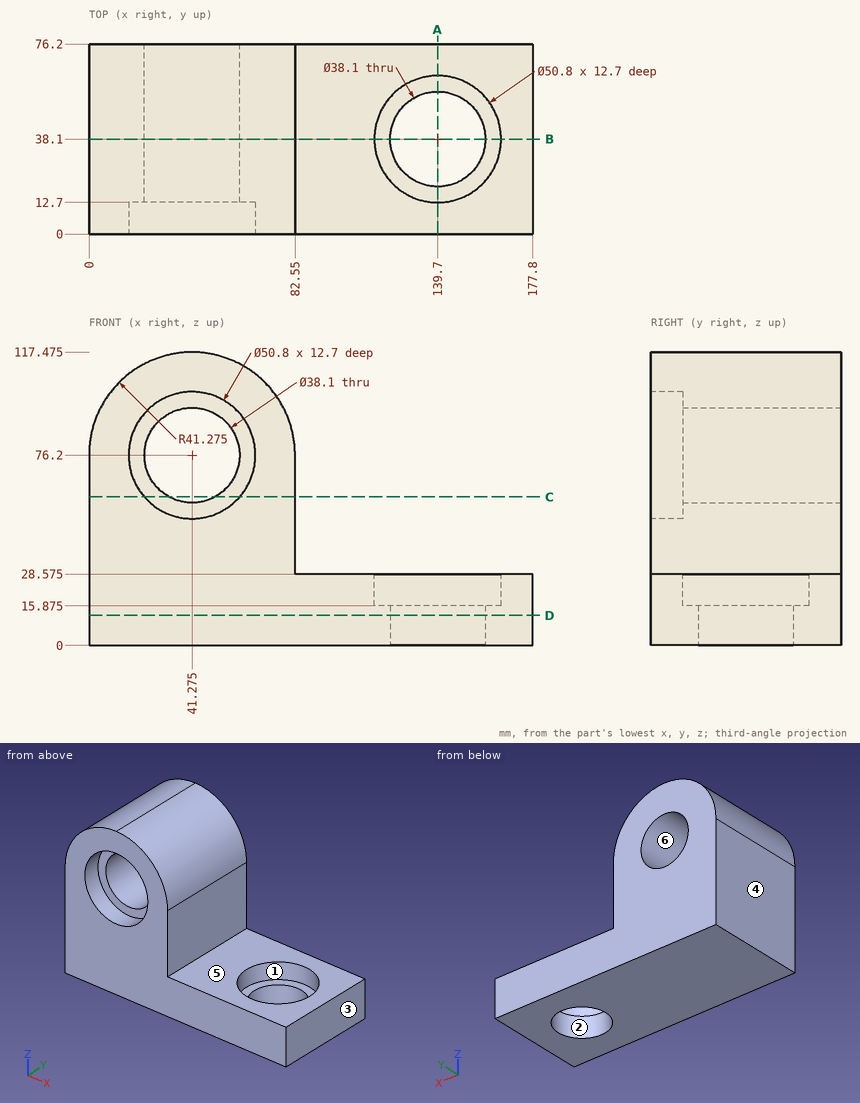
Print and shaded views of the part. All mm, measured from the part's lowest x, y and z. A direction names the side the tool comes from. Coordinates: 2 decimals unless noted, no trailing zeros. Loops run counter-clockwise (first coordinate to the right, second up) from the corner with the lowest first, then second, coordinate; pieces in that order, holes last. Notation, with made-up numbers: (19, -4.75) -> (45, -4.75) arc R24 ccw to (45, 23.25) -> close; hole circle Ø9 at (-31, 58.5). An arc over 180 degrees is marked (long way). Use one line per item in the form item = value. Start each with the question number.
(1) Cut at A-A on x = 139.7. Give the cut face in (y, z) (3 decimals), and give its area (3 significant figures).
(2) Flat gauge pins, fed straight in: pin 1 (5 mm diameter, centred on y = 12, z = 93, fed in from +X); pin 2 (1 mm diameter, centred on y = 9, z = 32, fed in from +X); pin 3 (23 mm diameter, centred on x = 139.7, y = 38.1, fed in from +Z); pin 4 (1.5 mm diameter, centred on y = 23, z = 80.5, fed in from +X). Where does each tip first touch, or does it go through?
(3) Cut at C-C on z = 59.5. Give the cut face in (x, y), and give its area (3 significant figures).
(4) Pull direction X, two halves, no side cores. Call the marked faces 1, 2, 3 and 4: pulls with the +X half, pulls with the -X half, needs draft (parallel to the pull), parting line crosses it, or undercut.
(5) Cut at B-B on y = 38.1. Give the cut face in (x, z) (3 decimals).
(6) Cut at D-D on z = 12. Give the cut face in (x, y).
(7) Probe probe 1 along Y at (x, z) = (140, 25); probe 2 along X at (y, z) = (4, 45); probe 3 along X at (y, z) = (38, 4). List the from-to ranges inside material, lowest first. Write a range as from..to.
(8) Tool access for the marked faces 5 and 6: list every direction of +Z, -Z, +X, -X, +Y, -Y with a clear straight run to the whole face (end or side of a thin tool).
Values:
q1.outline = (0, 0) -> (19.05, 0) -> (19.05, 15.875) -> (12.7, 15.875) -> (12.7, 28.575) -> (0, 28.575) -> close; (57.15, 0) -> (76.2, 0) -> (76.2, 28.575) -> (63.5, 28.575) -> (63.5, 15.875) -> (57.15, 15.875) -> close
q1.area = 927 mm2
q2.pin_1 = 79.99
q2.pin_2 = 82.55
q2.pin_3 = through
q2.pin_4 = 82.4
q3.outline = (0, 0) -> (22.14, 0) -> (22.14, 12.7) -> (32.11, 12.7) -> (32.11, 76.2) -> (0, 76.2) -> close; (50.44, 12.7) -> (60.41, 12.7) -> (60.41, 0) -> (82.55, 0) -> (82.55, 76.2) -> (50.44, 76.2) -> close
q3.area = 4,640 mm2
q4.face_1 = undercut
q4.face_2 = undercut
q4.face_3 = pulls with the +X half
q4.face_4 = pulls with the -X half
q5.outline = (0, 0) -> (120.65, 0) -> (120.65, 15.875) -> (114.3, 15.875) -> (114.3, 28.575) -> (82.55, 28.575) -> (82.55, 76.2) arc R41.275 ccw to (41.275, 117.475) arc R41.275 ccw to (0, 76.2) -> close; (158.75, 0) -> (177.8, 0) -> (177.8, 28.575) -> (165.1, 28.575) -> (165.1, 15.875) -> (158.75, 15.875) -> close; hole circle Ø38.1 at (41.275, 76.2)
q6.outline = (0, 0) -> (177.8, 0) -> (177.8, 76.2) -> (0, 76.2) -> close; hole circle Ø38.1 at (139.7, 38.1)
q7.probe_1 = 0..12.7, 63.5..76.2
q7.probe_2 = 0..82.55
q7.probe_3 = 0..120.65, 158.75..177.8
q8.face_5 = +Z, +X, +Y, -Y
q8.face_6 = +Y, -Y
